```python
from build123d import *

# Parameters (mm, degrees)
CYLINDER004_R     = 0.8
CYLINDER004_DEPTH = 5
CYLINDER006_R     = 2
CYLINDER006_DEPTH = 1.6
FILLET003_R       = 1
BOX006_W          = 25
BOX006_H          = 5
BOX006_DEPTH      = 1


with BuildPart() as cilindro004:
    # Cylinder004 → Cylinder004 (new body)
    with BuildSketch(Plane(origin=(-8, 104, -2), x_dir=(1, 0, 0), z_dir=(0, 0, 1))):
        Circle(CYLINDER004_R)
    extrude(amount=CYLINDER004_DEPTH)


with BuildPart() as fillet003:
    # Cylinder006 → Cylinder006 (new body)
    with BuildSketch(Plane(origin=(-8, 104, 0), x_dir=(1, 0, 0), z_dir=(0, 0, 1))):
        Circle(CYLINDER006_R)
    extrude(amount=CYLINDER006_DEPTH)

    # Fusion003: union Cilindro004
    add(cilindro004.part)

    # Fillet003
    fillet003_edges = [fillet003.edges().sort_by_distance(p)[0] for p in [
        (-8.8, 104, 1.6),
    ]]
    fillet(fillet003_edges, radius=FILLET003_R)


with BuildPart() as obj1:
    # Box006 → Box006 (new body)
    with BuildSketch(Plane(origin=(-30, 101.5, 0.55), x_dir=(1, 0, 0), z_dir=(0, 0, 1))):
        with Locations((12.5, 2.5)):
            Rectangle(BOX006_W, BOX006_H)
    extrude(amount=BOX006_DEPTH)

    # Fusion005: union Fillet003
    add(fillet003.part)


with BuildPart() as obj1_1:
    # Fusion005 placement: moved
    add(obj1.part.moved(Location((-5, 0, 0))))


solid = obj1_1.part
```
Work out the finished part from the listing and answer in its coordinate system (mm). A direction names the side the tool comes from. Give positions to 0.01 mm unless a question says otherwise; leave off trailing zeros. Order: outer loops, then holes, each group sorted by start corner. A loop starts at its lowest first (then second) coordinate and runs counter-clockwise, first axis right, second up. Notation, with made-up numbers: M 43.5,1.5 L 57.5,1.5 A11 ccw 57.5,15.5 Z; hole C -17.75,21.5 d4. An arc over 180 degrees is marked long. Return JSON: item names as keys, results as strings.
1) Section C-C, the plane z = -1.55 is taken. Write down the section's boundary in (x, y), plus the area to 3 significant figures.
Resolved:
{"outline": "C -13,104 d1.6", "area": "2.01 mm^2"}
2) Straight lines are drawn through the part: line 1 along Z through (x, y) = (-16.5, 105.8); line 2 along Y through (x, z) = (-14, 0.45); line 3 along Y through (x, z) = (-12.5, -0.6). For each, find the intervals that lie inside material, in ascending order. Write a range as [from, to].
Resolved:
{"line 1": "[0.55, 1.55]", "line 2": "[102.27, 105.73]", "line 3": "[103.38, 104.62]"}
3) Section A-A, the plane y = 104 is taken. Write down the section's boundary in (x, z).
Resolved:
{"outline": "M -35,0.55 L -15,0.55 L -15,0 L -13.8,0 L -13.8,-2 L -12.2,-2 L -12.2,0 L -11,0 L -11,0.55 L -10,0.55 L -10,1.55 L -11,1.55 L -11,1.6 L -11.2,1.6 A1 cw -12.2,2.6 L -12.2,3 L -13.8,3 L -13.8,2.6 A1 cw -14.8,1.6 L -15,1.6 L -15,1.55 L -35,1.55 Z"}
4) Each of these flat-tipped pins is pushed along its axis until it touches: pin 1 (1.5 mm diameter, centred on x = -28, z = -1, fed in from +Y); pin 2 (1 mm diameter, centred on x = -18.5, y = 104, fed in from +Z); pin 3 (1 mm diameter, centred on x = -31.5, y = 103.5, fed in from -Z). Where does it stop, or does it pass through?
Resolved:
{"pin 1": "through", "pin 2": "z = 1.55", "pin 3": "z = 0.55"}
5) A tool of negligible diameter and unlimited length cuts with its end or side. For faces 1 (the cylindrical face through (-13.59, 104.54, 2.8)), 2 (the cylindrical face through (-13.59, 104.54, -1.01)), 3 (the flat face through (-23, 106.5, 1)), from which of +Z, -Z, +X, -X, +Y, -Y can it reach the whole face along a straight path? Write none if from no direction.
Resolved:
{"face 1": "+Z", "face 2": "-Z", "face 3": "+Z, -Z, +X, -X, +Y"}
6) Section D-D, the plane x = -28 is taken. Write down the section's boundary in (y, z).
Resolved:
{"outline": "M 101.5,0.55 L 106.5,0.55 L 106.5,1.55 L 101.5,1.55 Z"}
7) Section B-B, the plane x = -13 is taken. Write down the section's boundary in (y, z), plus the area to 3 significant figures.
Resolved:
{"outline": "M 101.5,0.55 L 102,0.55 L 102,0 L 103.2,0 L 103.2,-2 L 104.8,-2 L 104.8,0 L 106,0 L 106,0.55 L 106.5,0.55 L 106.5,1.55 L 106,1.55 L 106,1.6 L 105.8,1.6 A1 cw 104.8,2.6 L 104.8,3 L 103.2,3 L 103.2,2.6 A1 cw 102.2,1.6 L 102,1.6 L 102,1.55 L 101.5,1.55 Z", "area": "13.3 mm^2"}
